Can you work these out from the model? Positions are in its coordinate system, mm. A direction names the side the tool comes from. Give positions to 0.01 mm unless a question says otherwise; leave off trailing zeros. Order: outer loops, then holes, each group sorted by start corner. A loop starts at its lowest first (then second) coordinate and runs counter-clockwise, first axis right, second up. Notation, with made-up numbers: M -39,10 L -14,10 A24 cw -14,49 Z; hole C -17.75,13 d2. An arc over 180 degrees is marked long. Write each question's results on one line, items separated by ' | '.
from build123d import *

# Parameters (mm, degrees)
SKETCH3_R           = 50.5
BOSS_EXTRUDE1_DEPTH = 40.5
SKETCH5_W           = 20
SKETCH5_H           = 130
CUT_EXTRUDE1_DEPTH  = 81
SKETCH9_R           = 4
CUT_EXTRUDE4_DEPTH  = 20
SKETCH10_R          = 42.5
CUT_EXTRUDE5_DEPTH  = 17
CHAMFER1_SIZE       = 1
CHAMFER2_SIZE       = 3
CUT_EXTRUDE8_START  = -13
SKETCH13_OUTSIDE_W  = 143.386
SKETCH13_OUTSIDE_H  = 166.386
SKETCH13_OUTSIDE_R  = 47.5
CUT_EXTRUDE8_DEPTH  = 10


with BuildPart() as part:
    # Sketch1 → Revolve1 (revolve)
    with BuildSketch(Plane.XY, mode=Mode.PRIVATE) as revolve1_sk:
        with BuildLine():
            Line((0, 0), (-61.5, 0))
            Line((-61.5, 0), (-61.5, 13))
            Line((-61.5, 13), (-45.5, 22.237604307))
            ThreePointArc((-45.5, 22.237604307), (-41.839745962, 25.897858345), (-40.5, 30.897858345))
            Line((-40.5, 30.897858345), (-40.5, 80))
            Line((-40.5, 80), (0, 80))
            Line((0, 80), (0, 0))
        make_face()
    revolve(revolve1_sk.sketch.rotate(Axis((0, 0, 0), (0, 1, 0)), 270), axis=Axis((0, 0, 0), (0, 1, 0)))

    # Sketch3 → Boss-Extrude1 (add, symmetric)
    with BuildSketch(Plane(origin=(0, 0, 0), x_dir=(0, 0, -1), z_dir=(1, 0, 0))):
        with Locations((0, 82.5)):
            Circle(SKETCH3_R)
    extrude(amount=BOSS_EXTRUDE1_DEPTH, both=True)

    # Sketch5 → Cut-Extrude1 (cut)
    with BuildSketch(Plane.XZ):
        with Locations((60, 0)):
            Rectangle(SKETCH5_W, SKETCH5_H)
        with Locations((-60, 0)):
            Rectangle(SKETCH5_W, SKETCH5_H)
    extrude(amount=-CUT_EXTRUDE1_DEPTH, mode=Mode.SUBTRACT)

    # Sketch6 → Cut-Revolve1 (revolve, cut)
    with BuildSketch(Plane.XY, mode=Mode.PRIVATE) as cut_revolve1_sk:
        Polygon((-35.5, 122.5), (-40.5, 122.5), (-40.5, 82.5), (40.5, 82.5), (40.5, 122.5), (35.5, 122.5), (35.5, 124.3), (32.8, 124.3), (32.8, 122.5), (19.8, 122.5), (19.8, 115), (-19.8, 115), (-19.8, 122.5), (-32.8, 122.5), (-32.8, 124.3), (-35.5, 124.3), align=None)
    revolve(cut_revolve1_sk.sketch.rotate(Axis((40.5, 82.5, 0), (1, 0, 0)), 90), axis=Axis((40.5, 82.5, 0), (1, 0, 0)), mode=Mode.SUBTRACT)

    # Sketch9 → Cut-Extrude4 (cut)
    with BuildSketch(Plane.XZ):
        with Locations(Location((38.183766184, 38.183766184, 0), (0, 0, 270))):
            Circle(SKETCH9_R)
        with Locations(Location((-38.183766184, 38.183766184, 0), (0, 0, 270))):
            Circle(SKETCH9_R)
        with Locations(Location((-38.183766184, -38.183766184, 0), (0, 0, 270))):
            Circle(SKETCH9_R)
        with Locations(Location((38.183766184, -38.183766184, 0), (0, 0, 270))):
            Circle(SKETCH9_R)
    extrude(amount=-CUT_EXTRUDE4_DEPTH, mode=Mode.SUBTRACT)

    # Sketch10 → Cut-Extrude5 (cut)
    with BuildSketch(Plane.XZ):
        with Locations(Location((0, 0, 0), (0, 0, 270))):
            Circle(SKETCH10_R)
    extrude(amount=-CUT_EXTRUDE5_DEPTH, mode=Mode.SUBTRACT)

    # Chamfer1
    # the kernel refuses this chamfer: 1 mm, written as the material it takes off along each edge
    with BuildSketch(Plane(origin=(-40.5, 82.5, 0), x_dir=(0, -1, 0), z_dir=(0, 0, 1))) as chamfer1_piece_1:
        Polygon((40 + CHAMFER1_SIZE, 0), (40, CHAMFER1_SIZE), (40, 0), align=None)
    revolve(axis=Axis((-40.5, 82.5, 0), (1, 0, 0)), revolution_arc=270, mode=Mode.SUBTRACT)
    with BuildSketch(Plane(origin=(40.5, 82.5, 0), x_dir=(0, -1, 0), z_dir=(0, 0, 1))) as chamfer1_piece_2:
        Polygon((40 + CHAMFER1_SIZE, 0), (40, -CHAMFER1_SIZE), (40, 0), align=None)
    revolve(axis=Axis((40.5, 82.5, 0), (1, 0, 0)), revolution_arc=270, mode=Mode.SUBTRACT)
    with BuildSketch(Plane(origin=(40.5, 82.5, 0), x_dir=(0, 0, 1), z_dir=(0, 1, 0))) as chamfer1_piece_3:
        Polygon((40 + CHAMFER1_SIZE, 0), (40, -CHAMFER1_SIZE), (40, 0), align=None)
    revolve(axis=Axis((40.5, 82.5, 0), (1, 0, 0)), revolution_arc=90, mode=Mode.SUBTRACT)
    with BuildSketch(Plane(origin=(-40.5, 82.5, 0), x_dir=(0, 0, 1), z_dir=(0, 1, 0))) as chamfer1_piece_4:
        Polygon((40 + CHAMFER1_SIZE, 0), (40, CHAMFER1_SIZE), (40, 0), align=None)
    revolve(axis=Axis((-40.5, 82.5, 0), (1, 0, 0)), revolution_arc=90, mode=Mode.SUBTRACT)

    # Chamfer2
    chamfer2_edges = [part.edges().sort_by_distance(p)[0] for p in [
        (0, 17, 42.5),
    ]]
    chamfer(chamfer2_edges, length=CHAMFER2_SIZE)

    # Sketch13 outside → Cut-Extrude8 (cut)
    with BuildSketch(Plane.XZ.offset(CUT_EXTRUDE8_START)):
        Rectangle(SKETCH13_OUTSIDE_W, SKETCH13_OUTSIDE_H)
        with Locations(Location((0, 0, 0), (0, 0, 270))):
            Circle(SKETCH13_OUTSIDE_R, mode=Mode.SUBTRACT)
    extrude(amount=-CUT_EXTRUDE8_DEPTH, mode=Mode.SUBTRACT)


solid = part.part
(1) Imagine slicing it at A-A, the plane x = 0. Write out the boundary of the cut face in (y, z), plus the area to 3 significant figures.
Data:
outline: M 0,-61.5 L 13,-61.5 L 13,-47.5 L 21.08,-47.5 L 22.24,-45.5 A10 cw 30.9,-40.5 L 52.33,-40.5 A50.5 ccw long 52.33,40.5 L 30.9,40.5 A10 cw 22.24,45.5 L 21.08,47.5 L 13,47.5 L 13,61.5 L 0,61.5 L 0,42.5 L 14,42.5 L 17,39.5 L 17,-39.5 L 14,-42.5 L 0,-42.5 Z; hole C 82.5,0 d65 | area: 7,040 mm2
(2) We'd pull the mould along X, two halves only. Please class faces 1 (the face through (10, 0, -42)), 2 (the face through (-34, 41, -5)), 3 (the face through (-25.861, 6.902, 33.727)), 4 (the face through (19.8, 49.7, -0.2)): +X half, -X half, draft (parallel to the pull), parting line (faces both ways), or undercut.
Data:
face 1: draft | face 2: undercut | face 3: undercut | face 4: +X half
(3) Will these pins go through, and if not, where does the flat tip stop? P1, Ø12, axis at x = -26, y = 37.5, coming from the +Z side; P2, Ø10, axis at y = 98.5, z = 42, coming from the -X side; P3, Ø6.5, axis at x = -38.18, z = 38.18, coming from the -Y side.
Data:
P1: stops at z = 35.22 | P2: stops at x = -40.5 | P3: stops at y = 46.03
(4) I need wall thicknesses on L1, parallel to Y at x = -7, z = 0; L2, parallel to Z at x = -33.4, y = 82.5; L3, parallel to Z at x = -24, y = 82. Which ranges of each line are inside material? Lowest first, please. Write a range as from..to.
Data:
L1: y = 17..50, 115..133 | L2: z = -50.5..-41.8, 41.8..50.5 | L3: z = -50.5..-40, 40..50.5
(5) For faces 5 (the face through (26.21, 42.84, -5.21)), 6 (the face through (-34.22, 6.41, -37.66)), 7 (the face through (-32.8, 104, -34)), 8 (the face through (40.5, 124, 0)), which set-ups out of +Z, -Z, +X, -X, +Y, -Y let a thin tool reach every point of the face, with its end or its side?
Data:
face 5: +X | face 6: -Y | face 7: none | face 8: +Z, -Z, +X, +Y
